Geometry: see drawing. Coordinates: mm, zero at the bounding-box minimum. Coordinates: 2 decimals unless noted, no trailing zeros. Loops run counter-clockwise (first coordinate to the right, second up) from the corner with the lowest first, then second, coordinate; pieces in that order, holes last. Notation, with made-up numbers: M -20.75,-34.5 L 3.25,-34.5 A22 cw 3.25,2.5 Z; hole C 57,21 d8. An arc over 180 degrees is marked long. One line per question, with ' | ' between items. Start each with the question number.
1. Ray query, probe 1 along Y at (x, z) = (73.25, 1); probe 2 along Y at (x, z) = (21.5, 2.7); probe 3 along X at (y, z) = (34.5, 0.35). Return the intervals inside material, ascending.
2. Section query C-C, the plane y = 5. Output: boundary loops of the cut face in (x, z), and give its area (3 significant figures).
3. Section query A-A, the plane x = 16.5. Output: boundary loops of the cut face in (y, z).
4. Section query B-B, the plane y = 11. Output: boundary loops of the cut face in (x, z), and give its area (3 significant figures).
5. Pin query (flat end, axial travel): P1, Ø3.5, axis at x = 73.25, y = 5, coming from the +Z side. Return the tip coordinate at first contact, or that it passes through.
6. Section query D-D, the plane z = 2.35. Output: boundary loops of the cut face in (x, y), and give its area (3 significant figures).
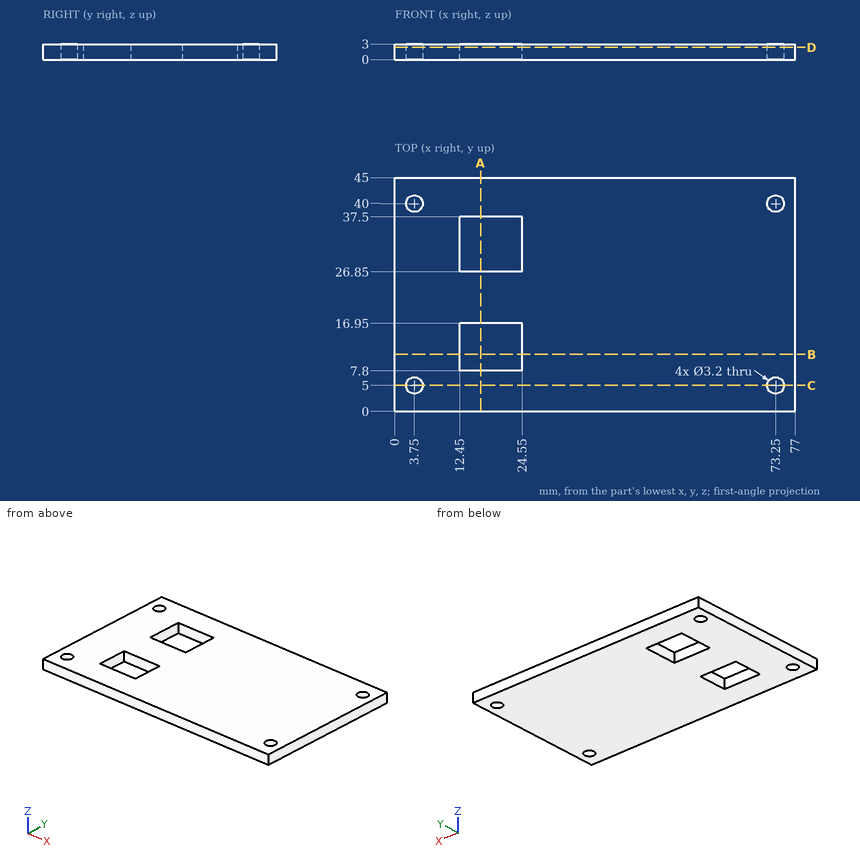
Taken from the geometry:
1) probe 1: 0 to 3.4, 6.6 to 38.4, 41.6 to 45 | probe 2: 0 to 7.8, 16.95 to 26.85, 37.5 to 45 | probe 3: 0 to 12.45, 24.55 to 77
2) outline: M 0,0 L 2.15,0 L 2.15,3 L 0,3 Z; M 5.35,0 L 71.65,0 L 71.65,3 L 5.35,3 Z; M 74.85,0 L 77,0 L 77,3 L 74.85,3 Z | area: 212 mm^2
3) outline: M 0,0 L 7.8,0 L 7.8,3 L 0,3 Z; M 16.95,0 L 26.85,0 L 26.85,3 L 16.95,3 Z; M 37.5,0 L 45,0 L 45,3 L 37.5,3 Z
4) outline: M 0,0 L 12.45,0 L 12.45,3 L 0,3 Z; M 24.55,0 L 77,0 L 77,3 L 24.55,3 Z | area: 195 mm^2
5) P1: z = 3
6) outline: M 0,0 L 77,0 L 77,45 L 0,45 Z; hole C 3.75,5 d3.2; hole C 3.75,40 d3.2; hole M 12.45,7.8 L 24.55,7.8 L 24.55,16.95 L 12.45,16.95 Z; hole M 12.45,26.85 L 24.55,26.85 L 24.55,37.5 L 12.45,37.5 Z; hole C 73.25,5 d3.2; hole C 73.25,40 d3.2 | area: 3,190 mm^2
